from build123d import *

# Parameters (mm, degrees)
SKETCH_1_W           = 40
SKETCH_1_H           = 30
EXTRUDE_1_DEPTH      = 5
SKETCH_2_W           = 5
SKETCH_2_H           = 30
EXTRUDE_2_DEPTH      = 20
SKETCH_3_W           = 20
SKETCH_3_H           = 30
EXTRUDE_3_DEPTH      = 5
SKETCH_4_W           = 15
SKETCH_4_H           = 30
CUT_EXTRUDE_1_DEPTH  = 5
SKETCH_5_R           = 1.5
CUT_EXTRUDE_2_DEPTH  = 5
SKETCH_6_R           = 3
CUT_EXTRUDE_3_DEPTH  = 2
SKETCH_7_W           = 15
SKETCH_7_H           = 30
CUT_EXTRUDE_4_DEPTH  = 10
SKETCH_8_W           = 5
SKETCH_8_H           = 30
EXTRUDE_4_DEPTH      = 20
SKETCH_10_W          = 30
SKETCH_10_H          = 30
EXTRUDE_5_DEPTH      = 3
SKETCH_11_R          = 1.5
CUT_EXTRUDE_6_DEPTH  = 13
SKETCH_12_R          = 2.9
CUT_EXTRUDE_7_DEPTH  = 6
SKETCH_14_W          = 8
SKETCH_14_H          = 20
EXTRUDE_6_DEPTH      = 20
CUT_EXTRUDE_8_DEPTH  = 4.2
SKETCH_16_R          = 1.5
CUT_EXTRUDE_9_DEPTH  = 14.2
SKETCH_17_R          = 2.9
CUT_EXTRUDE_10_DEPTH = 6
SKETCH_18_W          = 4
SKETCH_18_H          = 30
EXTRUDE_7_DEPTH      = 9.8
SKETCH_19_W          = 5
SKETCH_19_H          = 30
CUT_EXTRUDE_11_DEPTH = 26.2


with BuildPart() as part:
    # 草图1 → 凸台-拉伸1 (new body)
    with BuildSketch(Plane.XY):
        with Locations((-20, 15)):
            Rectangle(SKETCH_1_W, SKETCH_1_H)
    extrude(amount=EXTRUDE_1_DEPTH)

    # 草图2 → 凸台-拉伸2 (add)
    with BuildSketch(Plane.ZY.offset(40)):
        with Locations((2.5, 15)):
            Rectangle(SKETCH_2_W, SKETCH_2_H)
    extrude(amount=EXTRUDE_2_DEPTH)

    # 草图3 → 凸台-拉伸3 (add)
    with BuildSketch(Plane(origin=(0, 0, 0), x_dir=(-1, 0, 0), z_dir=(0, 0, -1))):
        with Locations((50, 15)):
            Rectangle(SKETCH_3_W, SKETCH_3_H)
    extrude(amount=EXTRUDE_3_DEPTH)

    # 草图4 → 切除-拉伸1 (cut)
    with BuildSketch(Plane.XY.offset(5)):
        with Locations((-52.5, 15)):
            Rectangle(SKETCH_4_W, SKETCH_4_H)
    extrude(amount=-CUT_EXTRUDE_1_DEPTH, mode=Mode.SUBTRACT)

    # 草图5 → 切除-拉伸2 (cut)
    with BuildSketch(Plane.XY):
        with Locations((-52.5, 5)):
            Circle(SKETCH_5_R)
        with Locations((-52.5, 25)):
            Circle(SKETCH_5_R)
    extrude(amount=-CUT_EXTRUDE_2_DEPTH, mode=Mode.SUBTRACT)

    # 草图6 → 切除-拉伸3 (cut)
    with BuildSketch(Plane.XY):
        with Locations((-52.5, 25)):
            Circle(SKETCH_6_R)
        with Locations((-52.5, 5)):
            Circle(SKETCH_6_R)
    extrude(amount=-CUT_EXTRUDE_3_DEPTH, mode=Mode.SUBTRACT)

    # 草图7 → 切除-拉伸4 (cut)
    with BuildSketch(Plane.XY):
        with Locations((-52.5, 15)):
            Rectangle(SKETCH_7_W, SKETCH_7_H)
    extrude(amount=-CUT_EXTRUDE_4_DEPTH, mode=Mode.SUBTRACT)

    # 草图8 → 凸台-拉伸4 (add)
    with BuildSketch(Plane(origin=(0, 0, -5), x_dir=(-1, 0, 0), z_dir=(0, 0, -1))):
        with Locations((42.5, 15)):
            Rectangle(SKETCH_8_W, SKETCH_8_H)
    extrude(amount=EXTRUDE_4_DEPTH)

    # 草图10 → 凸台-拉伸5 (add)
    with BuildSketch(Plane.ZY.offset(45)):
        with Locations((-10, 15)):
            Rectangle(SKETCH_10_W, SKETCH_10_H)
    extrude(amount=EXTRUDE_5_DEPTH)

    # 草图11 → 切除-拉伸6 (cut)
    with BuildSketch(Plane.ZY.offset(48)):
        with Locations((-15, 5)):
            Circle(SKETCH_11_R)
    extrude(amount=-CUT_EXTRUDE_6_DEPTH, mode=Mode.SUBTRACT)

    # 草图12 → 切除-拉伸7 (cut)
    with BuildSketch(Plane.ZY.offset(48)):
        with Locations((-15, 5)):
            Circle(SKETCH_12_R)
    extrude(amount=-CUT_EXTRUDE_7_DEPTH, mode=Mode.SUBTRACT)

    # 草图14 → 凸台-拉伸6 (add)
    with BuildSketch(Plane(origin=(0, 0, -25), x_dir=(-1, 0, 0), z_dir=(0, 0, -1))):
        with Locations((44, 20)):
            Rectangle(SKETCH_14_W, SKETCH_14_H)
    extrude(amount=EXTRUDE_6_DEPTH)

    # 草图15 → 切除-拉伸8 (cut)
    with BuildSketch(Plane(origin=(-40, 0, 0), x_dir=(0, 0, -1), z_dir=(1, 0, 0))):
        Polygon((45, 10), (25, 10), (25, 0), (18, 0), (18, 10), (18, 17), (45, 17), align=None)
    extrude(amount=-CUT_EXTRUDE_8_DEPTH, mode=Mode.SUBTRACT)

    # 草图16 → 切除-拉伸9 (cut)
    with BuildSketch(Plane.ZY.offset(48)):
        with Locations((-35, 20)):
            Circle(SKETCH_16_R)
    extrude(amount=-CUT_EXTRUDE_9_DEPTH, mode=Mode.SUBTRACT)

    # 草图17 → 切除-拉伸10 (cut)
    with BuildSketch(Plane.ZY.offset(48)):
        with Locations((-35, 20)):
            Circle(SKETCH_17_R)
    extrude(amount=-CUT_EXTRUDE_10_DEPTH, mode=Mode.SUBTRACT)

    # 草图18 → 凸台-拉伸7 (add)
    with BuildSketch(Plane(origin=(-40, 0, 0), x_dir=(0, 0, -1), z_dir=(1, 0, 0))):
        with Locations((2, 15)):
            Rectangle(SKETCH_18_W, SKETCH_18_H)
    extrude(amount=EXTRUDE_7_DEPTH)

    # 草图19 → 切除-拉伸11 (cut)
    with BuildSketch(Plane(origin=(0, 0, 0), x_dir=(0, 0, -1), z_dir=(1, 0, 0))):
        with Locations((-2.5, 15)):
            Rectangle(SKETCH_19_W, SKETCH_19_H)
    extrude(amount=-CUT_EXTRUDE_11_DEPTH, mode=Mode.SUBTRACT)


solid = part.part
Could you check a few things on this model? Use its own coordinates, in mm. A direction names the side the tool comes from. Coordinates: 2 decimals unless noted, no trailing zeros. Order: outer loops, then holes, each group sorted by start corner. A loop starts at its lowest first (then second) coordinate and runs counter-clockwise, first axis right, second up.
Q1. Thinking about a two-plate mould opening in Z: for faces 4 (the flat face through (-30.2, 15, -2)), 5 (the flat face through (-42, 18.8, -33.8)), 6 (the flat face through (-44, 22, -45)), which applies, released by +Z, released by -Z, zero draft, split by the parting line, or undercut?
Q2. Please list where these lines run through material, in increasing order: L1, parallel to Y at x = -44.8, z = -15; L2, parallel to Y at x = -40.85, z = -35; L3, parallel to Z at x = -37.5, y = 10.
Q3. Which directions (+Z, -Z, +X, -X, +Y, -Y) give clear straight access to the entire face, cutting with the end or side of a thin tool? Please do faces 1 (the cylindrical face through (-45.04, 18.89, -32.32)), 2 (the flat face through (-44.2, 12, -29)), 3 (the flat face through (-46, 10, -35)).
Q4. Suppose I cut it at C-C on x = -40.5. Please give me the cut outline in (y, z), and give its area (3 significant figures).
Q5. Suppose I cut it at B-B on y = 20. Please give me the cut outline in (x, z), and give its area (3 significant figures).
Q6. Suppose I cut it at A-A on z = -15. Please give me the cut outline in (x, y).
Q7. Suppose I cut it at D-D on z = -35. Please give me the cut outline in (x, y).
Q8. Will these pins go through, and if not, where does the flat tip stop? pin 1 (13.5 mm diameter, centred on y = 12, z = -38, fed in from +X); pin 2 (3.5 mm diameter, centred on x = -41.5, z = -35.5, fed in from -Y); pin 3 (8 mm diameter, centred on x = -30.5, y = 23, fed in from -Z).
Answer:
1. face 4: zero draft
1. face 5: undercut
1. face 6: released by -Z
2. L1: y = 0 to 2.1, 7.9 to 30
2. L2: y = 17 to 18.5, 21.5 to 30
2. L3: z = -4 to 5
3. face 1: -X
3. face 2: -Z, +X, -Y
3. face 3: -Z, +X, -X, -Y
4. outline: (0, -18) - (17, -18) - (17, -45) - (30, -45) - (30, 5) - (0, 5) - close; hole circle Ø3 at (5, -15); hole circle Ø3 at (20, -35)
4. area: 1,030 mm2
5. outline: (-48, -45) - (-40, -45) - (-40, -36.5) - (-42, -36.5) - (-42, -37.9) - (-48, -37.9) - close; (-48, -32.1) - (-42, -32.1) - (-42, -33.5) - (-40, -33.5) - (-40, -4) - (-30.2, -4) - (-30.2, 0) - (-26.2, 0) - (-26.2, 5) - (-48, 5) - close
5. area: 467 mm2
6. outline: (-48, 0) - (-40, 0) - (-40, 3.5) - (-42, 3.5) - (-42, 2.1) - (-48, 2.1) - close; (-48, 7.9) - (-42, 7.9) - (-42, 6.5) - (-40, 6.5) - (-40, 30) - (-48, 30) - close
7. outline: (-48, 10) - (-44.2, 10) - (-44.2, 17) - (-40, 17) - (-40, 18.5) - (-42, 18.5) - (-42, 17.1) - (-48, 17.1) - close; (-48, 22.9) - (-42, 22.9) - (-42, 21.5) - (-40, 21.5) - (-40, 30) - (-48, 30) - close
8. pin 1: stops at x = -40
8. pin 2: stops at y = 17
8. pin 3: stops at z = -4
